Work out the finished part from the listing and answer in its coordinate system (mm). Coordinates: 2 decimals unless noted, no trailing zeros. Write each loop counter-clockwise with the first axis right and the second up, starting at its lowest first coordinate (ties: lowest second). Pieces come first, ordered by that corner, then holes. Notation, with made-up numbers: (34, 18.5) - (91, 18.5) arc R29 ccw to (91, 52.5) - close; hole circle Ø9 at (4, 55.25). An arc over 180 degrees is marked (long way). Use one line per item in the form item = value. Start each with the question number.
Item 1: A cutting plane is placed at A-A (x = 80). Write down the section's boundary in (y, z).
Item 2: Consider probe 1 along Y at (x, z) = (-80, 5.5); probe 2 along Y at (x, z) = (82, 7.5); probe 3 along Y at (x, z) = (138.5, 1.5). Determine where each line is inside the solid, lowest interval first.
from build123d import *

# Parameters (mm, degrees)
ESQUISSE1_W              = 305
ESQUISSE1_H              = 305
BOSS_EXTRU_1_DEPTH       = 10
CONG_2_R                 = 15
ESQUISSE3_R              = 5
ENL_V_MAT_EXTRU_11_DEPTH = 10


with BuildPart() as part:
    # Esquisse1 → Boss.-Extru.1 (new body)
    with BuildSketch(Plane.XY):
        Rectangle(ESQUISSE1_W, ESQUISSE1_H)
    extrude(amount=BOSS_EXTRU_1_DEPTH)

    # Congé2
    cong_2_edges = [part.edges().sort_by_distance(p)[0] for p in [
        (-152.5, 152.5, 5),
        (152.5, 152.5, 5),
        (152.5, -152.5, 5),
        (-152.5, -152.5, 5),
    ]]
    fillet(cong_2_edges, radius=CONG_2_R)

    # Esquisse3 → Enlèv. mat.-Extru.11 (cut)
    with BuildSketch(Plane.XY.offset(10)):
        with Locations((80, 80)):
            Circle(ESQUISSE3_R)
        with Locations((80, -80)):
            Circle(ESQUISSE3_R)
        with Locations((-80, -80)):
            Circle(ESQUISSE3_R)
        with Locations((-80, 80)):
            Circle(ESQUISSE3_R)
    extrude(amount=-ENL_V_MAT_EXTRU_11_DEPTH, mode=Mode.SUBTRACT)


solid = part.part
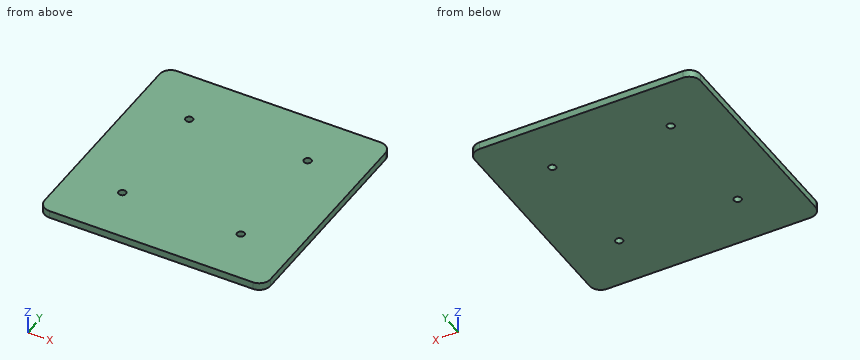
Answer:
q1.outline = (-152.5, 0) - (-85, 0) - (-85, 10) - (-152.5, 10) - close; (-75, 0) - (75, 0) - (75, 10) - (-75, 10) - close; (85, 0) - (152.5, 0) - (152.5, 10) - (85, 10) - close
q2.probe_1 = -152.5 to -85, -75 to 75, 85 to 152.5
q2.probe_2 = -152.5 to -84.58, -75.42 to 75.42, 84.58 to 152.5
q2.probe_3 = -152.47 to 152.47
